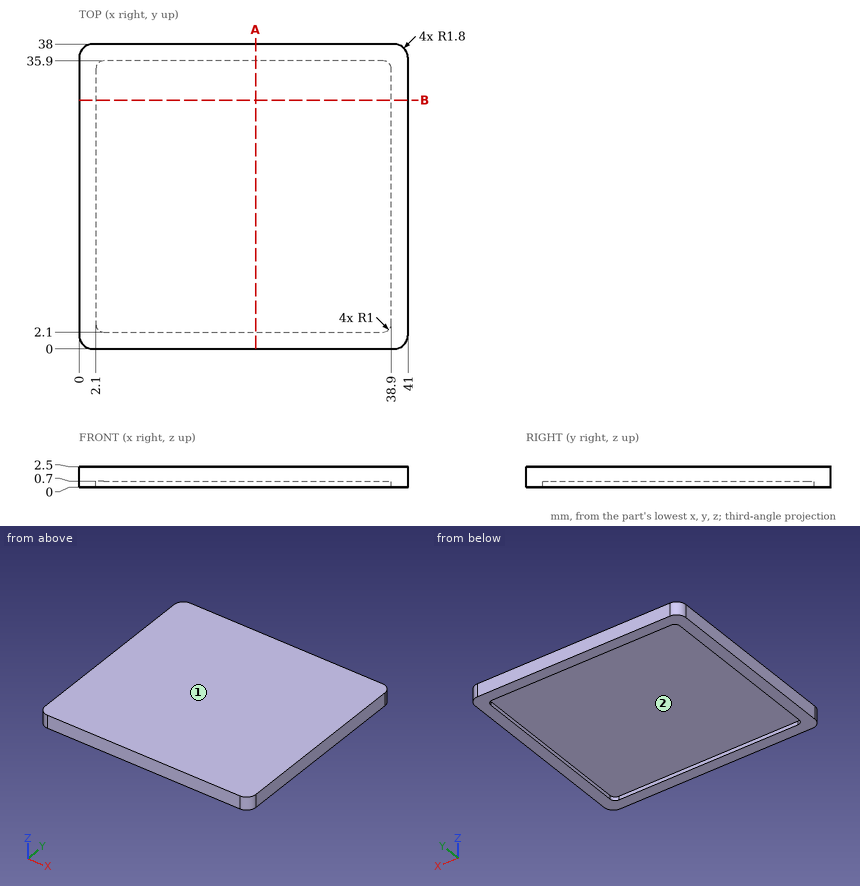
Source: three-view drawing plus pictorial views. Frame: mm from the lowest corner of the part. Coordinates: 2 decimals unless noted, no trailing zeros. Order: outer loops, then holes, each group sorted by start corner. A loop starts at its lowest first (then second) coordinate and runs counter-clockwise, first axis right, second up. Notation, with made-up numbers: M 10.5,64 L 26.5,64 A28 ccw 26.5,91 Z; hole C -14,-16 d1. An arc over 180 degrees is marked long. Write each question's results on one line, items separated by ' | '. Start each with the question number.
1. Section A-A, the plane x = 22. Return the cut outline in (y, z), then the cut area to 3 significant figures.
2. Draft query along X for the marked faces 1 and 2. Return one class per face: +X half, -X half, draft (parallel to the pull), parting line (faces both ways), or undercut.
3. Section B-B, the plane y = 31. Return the cut outline in (x, z), then the cut area to 3 significant figures.
4. Material intervals for L1, parallel to Y at x = 28, z = 0.65; L2, parallel to Z at x = 13, y = 8; L3, parallel to X at y = 3, z = 0.45, sorted ascending.
5. Pin query (flat end, axial travel): pin 1 (17 mm diameter, centred on x = 22.5, y = 14, fed in from -Z). Return the tip coordinate at first contact, or that it passes through.
Solution:
1) outline: M 0,0 L 2.1,0 L 2.1,0.7 L 35.9,0.7 L 35.9,0 L 38,0 L 38,2.5 L 0,2.5 Z | area: 71.3 mm²
2) face 1: draft | face 2: undercut
3) outline: M 0,0 L 2.1,0 L 2.1,0.7 L 38.9,0.7 L 38.9,0 L 41,0 L 41,2.5 L 0,2.5 Z | area: 76.7 mm²
4) L1: 0 to 2.1, 35.9 to 38 | L2: 0.7 to 2.5 | L3: 0 to 2.11, 38.89 to 41
5) pin 1: z = 0.7
